Design review of the part built by this model. Coordinates are the model's own, in mm. Face numbers are marked on the shaded views. A direction names the side the tool comes from. Coordinates: 2 decimals unless noted, no trailing zeros. Loops run counter-clockwise (first coordinate to the right, second up) from the corner with the lowest first, then second, coordinate; pieces in that order, holes last. Notation, with made-up numbers: (81, 44) -> (114, 44) arc R38 ccw to (114, 82) -> close; hole circle Ø9 at (10, 20.25). An arc over 180 degrees is marked (long way). Answer as a JSON object with one key per item and string values.
```python
from build123d import *

# Parameters (mm, degrees)
F1_DEPTH = 30
F3_DEPTH = 30.001
F5_DEPTH = 2


with BuildPart() as f1:
    # F0 (on Front) → F1 (new body)
    with BuildSketch(Plane.XZ):
        Polygon((-42.8425073624, 38.4018848052), (-42.8425073624, 0), (-15.4858445749, 0), (-15.4858445749, 30.194885969), align=None)
        Polygon((-66.6515186782, 45.5445881999), (-66.6515186782, 0), (-42.8425073624, 0), (-42.8425073624, 38.4018848052), align=None)
        Polygon((-81.502891345, 50), (-81.502891345, 0), (-66.6515186782, 0), (-66.6515186782, 45.5445881999), align=None)
        Polygon((-15.4858445749, 30.194885969), (-15.4858445749, 0), (18.497108655, 0), (18.497108655, 20), align=None)
    extrude(amount=F1_DEPTH)

    # F2 (on face) → F3 (cut, through all)
    with BuildSketch(Plane.XZ.offset(30)):
        Polygon((-66.4639249444, 45.4883100798), (-66.4639249444, 0), (-42.8256466985, 0), (-42.8256466985, 38.396826606), align=None)
        Polygon((-15.4689829797, 30.1898274904), (-15.4689829797, 0), (0, 0), (0, 25.5491325965), align=None)
    extrude(amount=-F3_DEPTH, mode=Mode.SUBTRACT)

    # F4 (on Front) → F5 (join)
    with BuildSketch(Plane.XZ):
        Polygon((18.5276474804, 49.7997477651), (-81.3374519348, 49.7997477651), (18.5276474804, 20.3182976693), align=None)
        Polygon((-81.3374519348, 0), (-81.3374519348, 49.7997477651), (-82.1342468262, 0), align=None)
        Polygon((18.5276474804, 20.3182976693), (-81.3374519348, 49.7997477651), (-81.3374519348, 0), (0, 0), (18.5276474804, 0), align=None)
    extrude(amount=-F5_DEPTH)


solid = f1.part
```
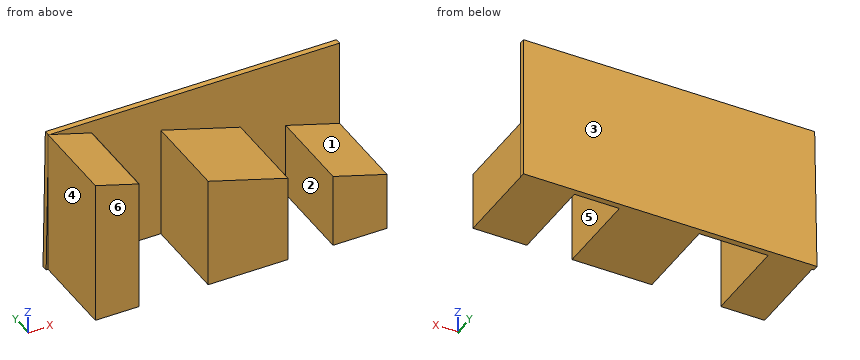
1) For the marked faces 1, 2 and 3, list the 3-axis set-ups (+Z, -Z, +X, -X, +Y, -Y) from which the entire face can be reached by the end or side of a thin tool; tool diameter is ignored.
Completed:
{"face 1": "+Z, +X, -Y", "face 2": "+Z, -Z, -Y", "face 3": "+Z, -Z, +X, -X, +Y"}
2) The part is to be moulded in two halves that separate along X. For the marked faces 4, 5 and 6, say which applies: pulls with the +X half, pulls with the -X half, needs draft (parallel to the pull), parting line crosses it, or undercut.
Completed:
{"face 4": "pulls with the -X half", "face 5": "undercut", "face 6": "needs draft"}
3) Wall thickness on probe 1 along X at (y, z) = (-1.5, 11); probe 2 along X at (y, z) = (-10, 43); probe 3 along Y at (x, z) = (-2.5, 45): over which ranges is each line inside the solid? List them lowest first.
Completed:
{"probe 1": "-81.5 to -66.46, -42.83 to -15.47, 0 to 18.5", "probe 2": "-81.5 to -66.46", "probe 3": "0 to 2"}
4) Add section C-C, the plane x = -8. Give the boundary of the cut face in (y, z), and give its area (3 significant figures).
Completed:
{"outline": "(0, 0) -> (2, 0) -> (2, 49.8) -> (0, 49.8) -> close", "area": "99.6 mm²"}
5) Clearance check with flat-ended pins moving along their axes: pin 1 Ø10 at (x, y) = (3.5, -15.5) entering from +Z; pin 2 Ø6 at (y, z) = (-15.5, 6) entering from +X; pin 3 Ø12 at (y, z) = (-6.5, 5.5) entering from -X. State where each tip first meets the part, or that it passes through.
Completed:
{"pin 1": "z = 25.55", "pin 2": "x = 18.5", "pin 3": "x = -81.5"}
6) Add section D-D, the plane z = 35. Give the boundary of the cut face in (x, y), and give its area (3 significant figures).
Completed:
{"outline": "(-81.57, 0) -> (-81.5, 0) -> (-81.5, -30) -> (-66.46, -30) -> (-66.46, 0) -> (-42.83, 0) -> (-42.83, -30) -> (-31.5, -30) -> (-31.5, 0) -> (18.53, 0) -> (18.53, 2) -> (-81.57, 2) -> close", "area": "991 mm²"}
7) Add section A-A, the plane y = -26. Give the boundary of the cut face in (x, z).
Completed:
{"outline": "(-81.5, 0) -> (-66.46, 0) -> (-66.46, 45.49) -> (-81.5, 50) -> close; (-42.83, 0) -> (-15.47, 0) -> (-15.47, 30.19) -> (-42.83, 38.4) -> close; (0, 0) -> (18.5, 0) -> (18.5, 20) -> (0, 25.55) -> close"}
